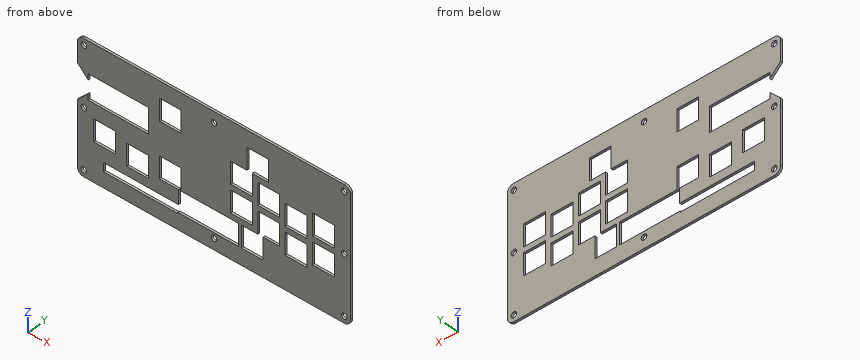
from build123d import *

# Parameters (mm, degrees)
SKETCH_1_R      = 2.55
SKETCH_1_W      = 20
SKETCH_1_H      = 20
EXTRUDE_1_DEPTH = 2


with BuildPart() as part:
    # 草图1 → 凸台-拉伸1 (new body)
    with BuildSketch(Plane(origin=(0, 0, 0), x_dir=(1, 0, 0), z_dir=(0, 1, 0))):
        with BuildLine():
            Line((15.755708479, 65.523244106), (15.755708479, 123.523244106))
            ThreePointArc((15.755708479, 123.523244106), (17.513067792, 127.765884793), (21.755708479, 129.523244106))
            Line((21.755708479, 129.523244106), (259.755708479, 129.523244106))
            ThreePointArc((259.755708479, 129.523244106), (263.998349166, 127.765884793), (265.755708479, 123.523244106))
            Line((265.755708479, 123.523244106), (265.755708479, 15.523244106))
            ThreePointArc((265.755708479, 15.523244106), (263.998349166, 11.280603419), (259.755708479, 9.523244106))
            Line((259.755708479, 9.523244106), (21.755708479, 9.523244106))
            ThreePointArc((21.755708479, 9.523244106), (17.513067792, 11.280603419), (15.755708479, 15.523244106))
            Line((15.755708479, 15.523244106), (15.755708479, 33.523244106))
            Line((15.755708479, 33.523244106), (25.755708479, 43.523244106))
            Line((25.755708479, 43.523244106), (25.755708479, 38.023244106))
            Line((25.755708479, 38.023244106), (80.755708479, 38.023244106))
            Line((80.755708479, 38.023244106), (80.755708479, 61.023244106))
            Line((80.755708479, 61.023244106), (25.755708479, 61.023244106))
            Line((25.755708479, 61.023244106), (25.755708479, 55.523244106))
            Line((25.755708479, 55.523244106), (15.755708479, 65.523244106))
        make_face()
        with Locations(Location((21.755708479, 123.523244106, 0), (0, 0, 270))):
            Circle(SKETCH_1_R, mode=Mode.SUBTRACT)
        with Locations(Location((259.755708479, 123.523244106, 0), (0, 0, 270))):
            Circle(SKETCH_1_R, mode=Mode.SUBTRACT)
        with Locations(Location((140.755708479, 119.523244106, 0), (0, 0, 270))):
            Circle(SKETCH_1_R, mode=Mode.SUBTRACT)
        with Locations(Location((21.755708479, 15.523244106, 0), (0, 0, 270))):
            Circle(SKETCH_1_R, mode=Mode.SUBTRACT)
        with Locations(Location((259.755708479, 15.523244106, 0), (0, 0, 270))):
            Circle(SKETCH_1_R, mode=Mode.SUBTRACT)
        with Locations(Location((140.755708479, 19.523244106, 0), (0, 0, 270))):
            Circle(SKETCH_1_R, mode=Mode.SUBTRACT)
        with Locations(Location((259.755708479, 69.523244106, 0), (0, 0, 270))):
            Circle(SKETCH_1_R, mode=Mode.SUBTRACT)
        with Locations(Location((21.755708479, 69.523244106, 0), (0, 0, 270))):
            Circle(SKETCH_1_R, mode=Mode.SUBTRACT)
        Polygon((107.755708479, 107.523244106), (39.755708479, 107.523244106), (39.755708479, 115.523244106), (107.755708479, 115.523244106), (107.755708479, 114.523244106), (108.255708479, 114.523244106), (163.255708479, 114.523244106), (163.255708479, 94.523244106), (110.755708479, 94.523244106), (110.755708479, 74.523244106), (90.755708479, 74.523244106), (90.755708479, 94.523244106), (108.255708479, 94.523244106), (108.255708479, 107.523244106), align=None, mode=Mode.SUBTRACT)
        with Locations((70.755708479, 89.523244106)):
            Rectangle(SKETCH_1_W, SKETCH_1_H, mode=Mode.SUBTRACT)
        with Locations((100.755708479, 34.523244106)):
            Rectangle(SKETCH_1_W, SKETCH_1_H, mode=Mode.SUBTRACT)
        with Locations((40.755708479, 84.523244106)):
            Rectangle(SKETCH_1_W, SKETCH_1_H, mode=Mode.SUBTRACT)
        Polygon((180.755708479, 94.523244106), (165.755708479, 94.523244106), (165.755708479, 114.523244106), (185.755708479, 114.523244106), (185.755708479, 94.523244106), (200.755708479, 94.523244106), (200.755708479, 74.523244106), (180.755708479, 74.523244106), align=None, mode=Mode.SUBTRACT)
        with Locations((165.755708479, 79.523244106)):
            Rectangle(SKETCH_1_W, SKETCH_1_H, mode=Mode.SUBTRACT)
        with Locations((215.755708479, 89.523244106)):
            Rectangle(SKETCH_1_W, SKETCH_1_H, mode=Mode.SUBTRACT)
        with Locations((240.755708479, 84.523244106)):
            Rectangle(SKETCH_1_W, SKETCH_1_H, mode=Mode.SUBTRACT)
        Polygon((170.755708479, 44.523244106), (155.755708479, 44.523244106), (155.755708479, 64.523244106), (175.755708479, 64.523244106), (175.755708479, 44.523244106), (190.755708479, 44.523244106), (190.755708479, 24.523244106), (170.755708479, 24.523244106), align=None, mode=Mode.SUBTRACT)
        with Locations((190.755708479, 59.523244106)):
            Rectangle(SKETCH_1_W, SKETCH_1_H, mode=Mode.SUBTRACT)
        with Locations((215.755708479, 64.523244106)):
            Rectangle(SKETCH_1_W, SKETCH_1_H, mode=Mode.SUBTRACT)
        with Locations((240.755708479, 59.523244106)):
            Rectangle(SKETCH_1_W, SKETCH_1_H, mode=Mode.SUBTRACT)
    extrude(amount=EXTRUDE_1_DEPTH)


solid = part.part
Here's how the part is built. I have some questions about the finished solid (model axes, mm). Give positions to 0.01 mm unless a question says otherwise; leave off trailing zeros. Write each loop counter-clockwise with the first axis right and the second up, starting at its lowest first coordinate (ties: lowest second). Pieces come first, ordered by that corner, then holes. Notation, with made-up numbers: (49.25, -23.75) -> (100.25, -23.75) arc R12 cw to (100.25, -7.75) -> close; hole circle Ø11 at (-20, 60.25). An arc over 180 degrees is marked (long way). Use one line per item in the form item = value. Start each with the question number.
1. Will these pins go through, and if not, where does the flat tip stop? pin 1 Ø12 at (x, z) = (167, -63) entering from -Y; pin 2 Ø0.6 at (y, z) = (1, -34.5) entering from -X; pin 3 Ø1 at (x, z) = (81, -109.5) entering from +Y.
2. Imagine slicing it at D-D on x = 96.5. List the corners of the cut face in (y, z) for me.
3. If I drill on L1, parallel to Z at x = 193.5, y = 0.9; L2, parallel to X at y = 0.5, z = -44; L3, parallel to X at y = 0.6, z = -112, over which ranges is the centre line in solid material (lowest first)?
4. Imagine slicing it at A-A on x = 66.5. List the corners of the cut face in (y, z) for me, plus the area to 3 significant figures.
5. Imagine slicing it at C-C on x = 126. List the corners of the cut face in (y, z) for me.
6. Imagine slicing it at B-B on z = -110.5. List the corners of the cut face in (x, y) for me, plus the area to 3 significant figures.
Entries:
q1.pin_1 = 0
q1.pin_2 = 16.43
q1.pin_3 = through
q2.outline = (0, -129.52) -> (2, -129.52) -> (2, -115.52) -> (0, -115.52) -> close; (0, -107.52) -> (2, -107.52) -> (2, -94.52) -> (0, -94.52) -> close; (0, -74.52) -> (2, -74.52) -> (2, -44.52) -> (0, -44.52) -> close; (0, -24.52) -> (2, -24.52) -> (2, -9.52) -> (0, -9.52) -> close
q3.L1 = -129.52 to -94.52, -74.52 to -69.52, -49.52 to -9.52
q3.L2 = 80.76 to 90.76, 110.76 to 170.76, 190.76 to 265.76
q3.L3 = 15.76 to 39.76, 163.26 to 165.76, 185.76 to 265.76
q4.outline = (0, -129.52) -> (2, -129.52) -> (2, -115.52) -> (0, -115.52) -> close; (0, -107.52) -> (2, -107.52) -> (2, -99.52) -> (0, -99.52) -> close; (0, -79.52) -> (2, -79.52) -> (2, -61.02) -> (0, -61.02) -> close; (0, -38.02) -> (2, -38.02) -> (2, -9.52) -> (0, -9.52) -> close
q4.area = 138 mm²
q5.outline = (0, -129.52) -> (2, -129.52) -> (2, -114.52) -> (0, -114.52) -> close; (0, -94.52) -> (2, -94.52) -> (2, -9.52) -> (0, -9.52) -> close
q6.outline = (15.76, 0) -> (39.76, 0) -> (39.76, 2) -> (15.76, 2) -> close; (163.26, 0) -> (165.76, 0) -> (165.76, 2) -> (163.26, 2) -> close; (185.76, 0) -> (265.76, 0) -> (265.76, 2) -> (185.76, 2) -> close
q6.area = 213 mm²
